Verification items for the finished model (mm, model axes). Face numbers are marked on the shaded views. A direction names the side the tool comes from. Round coordinates to 2 decimals unless told otherwise and drop trailing zeros. Order: outer loops, then holes, each group sorted by start corner. A loop starts at its lowest first (then second) coordinate and runs counter-clockwise, first axis right, second up. Notation, with made-up numbers: M -18.5,-12.75 L -2.5,-12.75 A16 cw -2.5,5.25 Z; hole C -9,56.25 d11. An arc over 180 degrees is marked long. Answer as a JSON object with one key per item and string values. Group by question number.
```python
from build123d import *

# Parameters (mm, degrees)
SM_BASE_FLANGE_1_DEPTH   = 13
HOLE_WIZARD_1_AT_2_COUNT = 2
HOLE_WIZARD_1_AT_2_PITCH = 18.5
HOLE_WIZARD_5_0_5_1_D    = 5
FILLET_1_R               = 5


# Sheet-metal steps are written as plain solids
with BuildPart() as part:
    # Sketch 1 → 基体-法兰1 (new, symmetric)
    with BuildSketch(Plane.XY):
        with BuildLine():
            Line((-16, 0), (15.647346039, 0))
            ThreePointArc((15.647346039, 0), (15.994642394, -0.030384494), (16.331386325, -0.120614758))
            Line((16.331386325, -0.120614758), (31, -5.459553514))
            Line((31, -5.459553514), (30.657979857, -6.399246135))
            Line((30.657979857, -6.399246135), (15.989366182, -1.060307379))
            ThreePointArc((15.989366182, -1.060307379), (15.820994216, -1.015192247), (15.647346039, -1))
            Line((15.647346039, -1), (-16, -1))
            Line((-16, -1), (-16, 0))
        make_face()
    extrude(amount=SM_BASE_FLANGE_1_DEPTH, both=True)

    # 草图6 → 打孔尺寸(%根据十字)槽沉头木螺钉的类型1 (revolve, cut)
    with BuildSketch(Plane(origin=(11, 0, 9.25), x_dir=(0, 0, 1), z_dir=(1, 0, 0))):
        Polygon((0, 0), (0, 1), (1.7, 1), (1.7, 1.6), (3.3, 0), align=None)
    hole_wizard_1 = revolve(axis=Axis((11, 6.35, 9.25), (0, -1, 0)), mode=Mode.SUBTRACT)

    # 打孔尺寸(%根据十字)槽沉头木螺钉的类型1 at 2: 打孔尺寸(%根据十字)槽沉头木螺钉的类型1 ×2
    with Locations(*[(0, 0, -i * HOLE_WIZARD_1_AT_2_PITCH) for i in range(1, HOLE_WIZARD_1_AT_2_COUNT)]):
        add(hole_wizard_1, mode=Mode.SUBTRACT)

    # Ø5.0 (5) 直径孔1 (through all)
    with Locations(Plane(origin=(0, 0, 0), x_dir=(1, 0, 0), z_dir=(0, 1, 0))):
        with Locations((-7.5, -7.3), (-7.5, 7.3)):
            Hole(HOLE_WIZARD_5_0_5_1_D / 2)

    # 圆角1
    fillet_1_edges = [part.edges().sort_by_distance(p)[0] for p in [
        (-16, -0.5, 13),
        (30.828989928, -5.929399824, 13),
        (-16, -0.5, -13),
        (30.828989928, -5.929399824, -13),
    ]]
    fillet(fillet_1_edges, radius=FILLET_1_R)


solid = part.part
```
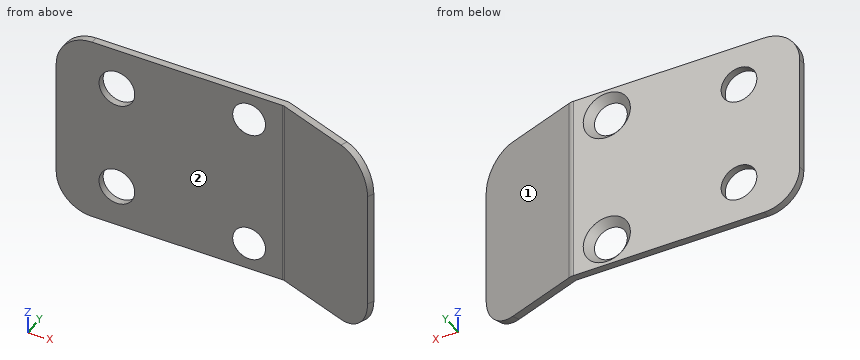
Q1. Cross-section at A-A, the plane x = -7.5. Record the cut outline in (y, z).
Q2. Thickness scan on line 1 (Z direction, x = -7.5, y = -0.5); line 2 (Z direction, x = -9.5, y = -0.5); line 3 (Y direction, x = -3.5, z = 5.75). Record the ranges inside material, lowest first. Write a range as from..to.
Q3. Cross-section at B-B, the plane z = -2.75. Record the cut outline in (x, y).
Q4. Gauge pin test, flat end, axial feed: pin 1 Ø4 at (x, z) = (8.5, -5.5) entering from -Y. Record the tip position at first contact, or that the pin passes through.
Q5. Cross-section at D-D, the plane x = 11. Record the cut outline in (y, z), then the cut area to 3 significant figures.
Q6. Cross-section at C-C, the plane z = 9.25. Record the cut outline in (x, y), then the cut area to 3 significant figures.
Q7. Tool access check on the marked faces 1 and 2. Record the directions out of +Z, -Z, +X, -X, +Y, -Y that give a thin tool (end or side, any length) a straight path to the whole face; none if there is none.
Conclusion:
{
 "1": {"outline": "M -1,-13 L 0,-13 L 0,-9.8 L -1,-9.8 Z; M -1,-4.8 L 0,-4.8 L 0,4.8 L -1,4.8 Z; M -1,9.8 L 0,9.8 L 0,13 L -1,13 Z"},
 "2": {"line 1": "-13..-9.8, -4.8..4.8, 9.8..13", "line 2": "-13..-8.8, -5.8..5.8, 8.8..13", "line 3": "-1..0"},
 "3": {"outline": "M -16,-1 L 15.65,-1 A1 cw 15.99,-1.06 L 30.66,-6.4 L 31,-5.46 L 16.33,-0.12 A2 ccw 15.65,0 L -16,0 Z"},
 "4": {"pin 1": "y = -1"},
 "5": {"outline": "M -1,-13 L 0,-13 L 0,-12.55 L -1,-11.55 Z; M -1,-6.95 L 0,-5.95 L 0,5.95 L -1,6.95 Z; M -1,11.55 L 0,12.55 L 0,13 L -1,13 Z", "area": "14.8 mm2"},
 "6": {"outline": "M -15.84,-1 L -9.06,-1 L -9.06,0 L -15.84,0 Z; M -5.94,-1 L 8.7,-1 L 7.7,0 L -5.94,0 Z; M 13.3,-1 L 15.65,-1 A1 cw 15.99,-1.06 L 30.51,-6.34 L 30.85,-5.41 L 16.33,-0.12 A2 ccw 15.65,0 L 14.3,0 Z", "area": "38.7 mm2"},
 "7": {"face 1": "+Z, -Z, +X, +Y", "face 2": "+Z, -Z, -X, -Y"}
}
